```python
from build123d import *

# Parameters (mm, degrees)
SKETCH1_R                        = 215.9
SKETCH1_R_2                      = 177.8
BOSS_EXTRUDE1_DEPTH              = 4.7498
BOSS_EXTRUDE2_DEPTH              = 4.7498
FILLET2_R                        = 12.7
FILLET3_R                        = 11.43
F_1_4_CLEARANCE_HOLE1_AT_2_COUNT = 2
F_1_4_CLEARANCE_HOLE1_AT_2_PITCH = 34.29
CIRPATTERN1_COUNT                = 4
FILLET2_OF_CIRPATTERN1_R         = 12.7
FILLET3_OF_CIRPATTERN1_R         = 11.43
SKETCH6_R                        = 9.525
CUT_EXTRUDE1_DEPTH               = 4.7498
CIRPATTERN2_COUNT                = 4


with BuildPart() as part:
    # Sketch1 → Boss-Extrude1 (new body)
    with BuildSketch(Plane(origin=(0, 0, 0), x_dir=(1, 0, 0), z_dir=(0, 1, 0))):
        Circle(SKETCH1_R)
        Circle(SKETCH1_R_2, mode=Mode.SUBTRACT)
    extrude(amount=BOSS_EXTRUDE1_DEPTH)

    # Sketch3 → Boss-Extrude2 (add)
    with BuildSketch(Plane(origin=(0, 0, 0), x_dir=(1, 0, 0), z_dir=(0, 1, 0))):
        with BuildLine():
            Line((-22.450640303, 176.376894037), (0, 153.926253734))
            Line((0, 153.926253734), (22.450640303, 176.376894037))
            ThreePointArc((22.450640303, 176.376894037), (0, 177.8), (-22.450640303, 176.376894037))
        make_face()
    boss_extrude2 = extrude(amount=BOSS_EXTRUDE2_DEPTH)

    # Fillet2
    fillet2_edges = [part.edges().sort_by_distance(p)[0] for p in [
        (22.450640303, 2.3749, -176.376894037),
        (-22.450640303, 2.3749, -176.376894037),
    ]]
    fillet(fillet2_edges, radius=FILLET2_R)

    # Fillet3
    fillet3_edges = [part.edges().sort_by_distance(p)[0] for p in [
        (0, 2.3749, -153.926253734),
    ]]
    fillet(fillet3_edges, radius=FILLET3_R)

    # Sketch5 → 1/4 Clearance Hole1 (revolve, cut)
    with BuildSketch(Plane(origin=(0, 4.7498, -170.090714752), x_dir=(0, 0, 1), z_dir=(1, 0, 0))):
        Polygon((0, 0), (0, 12.189827343), (3.3782, 10.16), (3.3782, 0), align=None)
    f_1_4_clearance_hole1 = revolve(axis=Axis((0, 11.0998, -170.090714752), (0, -1, 0)), mode=Mode.SUBTRACT)

    # 1/4 Clearance Hole1 at 2: 1/4 Clearance Hole1 ×2
    with Locations(*[(0, 0, -i * F_1_4_CLEARANCE_HOLE1_AT_2_PITCH) for i in range(1, F_1_4_CLEARANCE_HOLE1_AT_2_COUNT)]):
        add(f_1_4_clearance_hole1, mode=Mode.SUBTRACT)

    # CirPattern1: Boss-Extrude2, 1/4 Clearance Hole1 ×4 about axis
    cirpattern1_axis = Axis((0, 0, 0), (0, 1, 0))
    for i in range(1, CIRPATTERN1_COUNT):
        add(boss_extrude2.rotate(cirpattern1_axis, i * 360 / CIRPATTERN1_COUNT))
        add(f_1_4_clearance_hole1.rotate(cirpattern1_axis, i * 360 / CIRPATTERN1_COUNT), mode=Mode.SUBTRACT)

    # CirPattern1 copy 1 sketch → CirPattern1 copy 1 (revolve, cut)
    with BuildSketch(Plane(origin=(-204.380714752, 4.7498, 0), x_dir=(1, 0, 0), z_dir=(0, 0, -1))):
        Polygon((0, 0), (0, 12.189827343), (3.3782, 10.16), (3.3782, 0), align=None)
    revolve(axis=Axis((-204.380714752, 11.0998, 0), (0, -1, 0)), mode=Mode.SUBTRACT)

    # CirPattern1 copy 2 sketch → CirPattern1 copy 2 (revolve, cut)
    with BuildSketch(Plane(origin=(0, 4.7498, 204.380714752), x_dir=(0, 0, -1), z_dir=(-1, 0, 0))):
        Polygon((0, 0), (0, 12.189827343), (3.3782, 10.16), (3.3782, 0), align=None)
    revolve(axis=Axis((0, 11.0998, 204.380714752), (0, -1, 0)), mode=Mode.SUBTRACT)

    # CirPattern1 copy 3 sketch → CirPattern1 copy 3 (revolve, cut)
    with BuildSketch(Plane(origin=(204.380714752, 4.7498, 0), x_dir=(-1, 0, 0), z_dir=(0, 0, 1))):
        Polygon((0, 0), (0, 12.189827343), (3.3782, 10.16), (3.3782, 0), align=None)
    revolve(axis=Axis((204.380714752, 11.0998, 0), (0, -1, 0)), mode=Mode.SUBTRACT)

    # Fillet2 of CirPattern1
    fillet2_of_cirpattern1_edges = [part.edges().sort_by_distance(p)[0] for p in [
        (-176.376894037, 2.3749, -22.450640303),
        (-176.376894037, 2.3749, 22.450640303),
        (-22.450640303, 2.3749, 176.376894037),
        (22.450640303, 2.3749, 176.376894037),
        (176.376894037, 2.3749, 22.450640303),
        (176.376894037, 2.3749, -22.450640303),
    ]]
    fillet(fillet2_of_cirpattern1_edges, radius=FILLET2_OF_CIRPATTERN1_R)

    # Fillet3 of CirPattern1
    fillet3_of_cirpattern1_edges = [part.edges().sort_by_distance(p)[0] for p in [
        (-153.926253734, 2.3749, 0),
        (0, 2.3749, 153.926253734),
        (153.926253734, 2.3749, 0),
    ]]
    fillet(fillet3_of_cirpattern1_edges, radius=FILLET3_OF_CIRPATTERN1_R)

    # Sketch6 → Cut-Extrude1 (cut)
    with BuildSketch(Plane(origin=(0, 4.7498, 0), x_dir=(1, 0, 0), z_dir=(0, 1, 0))):
        with Locations((-139.193969877, 139.193969877)):
            Circle(SKETCH6_R)
    cut_extrude1 = extrude(amount=-CUT_EXTRUDE1_DEPTH, mode=Mode.SUBTRACT)

    # CirPattern2: Cut-Extrude1 ×4 about axis
    cirpattern2_axis = Axis((0, 0, 0), (0, 1, 0))
    for i in range(1, CIRPATTERN2_COUNT):
        add(cut_extrude1.rotate(cirpattern2_axis, i * 360 / CIRPATTERN2_COUNT), mode=Mode.SUBTRACT)


solid = part.part
```
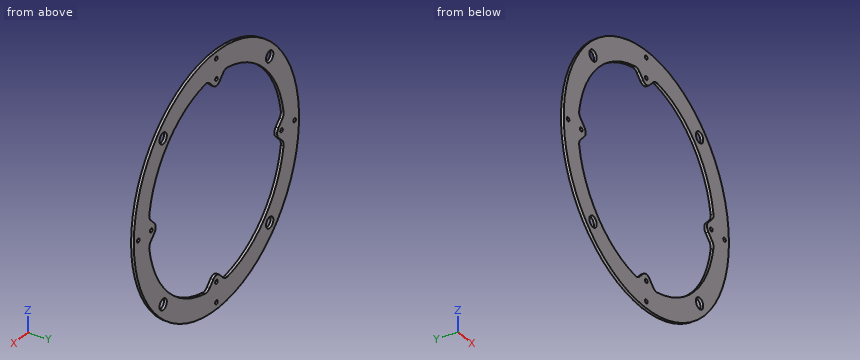
Here's how the part is built. I have some questions about the finished solid (model axes, mm). Round coordinates to 2 decimals unless told otherwise and drop trailing zeros. Order: outer loops, then holes, each group sorted by start corner. A loop starts at its lowest first (then second) coordinate and runs counter-clockwise, first axis right, second up. Notation, with made-up numbers: M 47.5,28 L 72.5,28 A24 ccw 72.5,54 Z; hole C 55,-26.75 d6. An arc over 180 degrees is marked long. Use CSV: the item, a comma, the result in double quotes.
1) I'm going to push a flat-ended pin straight in: P1, Ø1.5, axis at y = 2, z = -113.5, coming from the -X side. Where does the tip first touch, or does it pass through?
Taken from the geometry:
P1,"x = -184.12"
2) I want a section at A-A (x = 72.5). List the corners of the cut face in (y, z) for me.
Taken from the geometry:
outline,"M 0,-203.36 L 4.75,-203.36 L 4.75,-162.35 L 0,-162.35 Z; M 0,162.35 L 4.75,162.35 L 4.75,203.36 L 0,203.36 Z"
3) I want a section at C-C (y = 0.85). Count the separate pieces of the cut face and the enclosed holes in it, then the cut area to 3 significant figures.
Taken from the geometry:
separate pieces,"1"
enclosed holes,"13"
area,"47,800 mm^2"
4) I want a section at B-B (z = -114). List the corners of the cut face in (x, y) for me.
Taken from the geometry:
outline,"M -183.35,0 L -136.44,0 L -136.44,4.75 L -183.35,4.75 Z; M 136.44,0 L 183.35,0 L 183.35,4.75 L 136.44,4.75 Z"
5) I need wall thicknesses on line 1 along Z through (x, y) = (0, 2.2); line 2 along X through (y, z) = (1.25, 35.5); line 3 along X through (y, z) = (3.85, 92.5). Which ranges of each line are inside material? Lowest first, please. Write a range as [from, to].
Taken from the geometry:
line 1,"[-215.9, -207.76], [-201, -173.47], [-166.71, -158.66], [158.66, 166.71], [173.47, 201], [207.76, 215.9]"
line 2,"[-212.96, -174.22], [174.22, 212.96]"
line 3,"[-195.08, -151.84], [151.84, 195.08]"
